```python
from build123d import *

# Parameters (mm, degrees)
EXTRUDE_1_DEPTH   = 2
HOLE_WIZARD_M81_D = 9
CHAMFER_1_SIZE    = 2


with BuildPart() as part:
    # Эскиз1 → Бобышка-Вытянуть1 (new body)
    with BuildSketch(Plane(origin=(0, 0, 0), x_dir=(1, 0, 0), z_dir=(0, 0, -1))):
        Polygon((0, 0), (0, 90), (90, 90), (90, 45), (45, 45), (45, 0), align=None)
    extrude(amount=EXTRUDE_1_DEPTH)

    # Отверстие с зазором M81 (through all)
    with Locations(Plane(origin=(0, 0, -2), x_dir=(1, 0, 0), z_dir=(0, 0, -1))):
        with Locations((22.5, 67.5), (22.5, 22.5), (67.5, 67.5)):
            Hole(HOLE_WIZARD_M81_D / 2)

    # Фаска1
    chamfer_1_edges = [part.edges().sort_by_distance(p)[0] for p in [
        (0, 0, -1),
        (0, -90, -1),
        (90, -90, -1),
        (90, -45, -1),
        (45, 0, -1),
    ]]
    chamfer(chamfer_1_edges, length=CHAMFER_1_SIZE)


solid = part.part
```
Verification items for the finished model (mm, model axes). A direction names the side the tool comes from. Round coordinates to 2 decimals unless told otherwise and drop trailing zeros. Loops run counter-clockwise (first coordinate to the right, second up) from the corner with the lowest first, then second, coordinate; pieces in that order, holes last. Notation, with made-up numbers: (33, -29.75) -> (89, -29.75) arc R11 cw to (89, -11.75) -> close; hole circle Ø10 at (40, 53). An arc over 180 degrees is marked (long way). Answer as a JSON object with one key per item and string values.
Q1. Draft check along Y on faces 3 (the flat face through (44, -1, -1)), 4 (the cylindrical face through (25.82, -25.54, -0.99)), 5 (the flat face through (45, -24, -1)). Enter one of: pulls with the +Y half, pulls with the -Y half, needs draft (parallel to the pull), parting line crosses it, or undercut.
Data:
{"face 3": "pulls with the +Y half", "face 4": "undercut", "face 5": "needs draft"}
Q2. Section check B-B (x = 67.5). Record the boundary of the cut face in (y, z), then the cut area to 3 significant figures.
Data:
{"outline": "(-90, -2) -> (-72, -2) -> (-72, 0) -> (-90, 0) -> close; (-63, -2) -> (-45, -2) -> (-45, 0) -> (-63, 0) -> close", "area": "72.0 mm2"}
Q3. Section check D-D (z = -1.2). Record the boundary of the cut face in (x, y), then the cut area to 3 significant figures.
Data:
{"outline": "(0, -88) -> (2, -90) -> (88, -90) -> (90, -88) -> (90, -47) -> (88, -45) -> (45, -45) -> (45, -2) -> (43, 0) -> (2, 0) -> (0, -2) -> close; hole circle Ø9 at (22.5, -67.5); hole circle Ø9 at (22.5, -22.5); hole circle Ø9 at (67.5, -67.5)", "area": "5,870 mm2"}
Q4. Section check C-C (y = -22.5). Record the boundary of the cut face in (x, z).
Data:
{"outline": "(0, -2) -> (18, -2) -> (18, 0) -> (0, 0) -> close; (27, -2) -> (45, -2) -> (45, 0) -> (27, 0) -> close"}
Q5. Access from +Z, -Z, +X, -X, +Y, -Y to the whole of each face (thin tool, end or side, straight path). Record for faces 1 (the flat face through (1, -89, -1)), 2 (the flat face through (67, -45, -1)).
Data:
{"face 1": "+Z, -Z, -X, -Y", "face 2": "+Z, -Z, +X, +Y"}
Q6. Section check A-A (x = 22.5). Record the boundary of the cut face in (y, z), then the cut area to 3 significant figures.
Data:
{"outline": "(-90, -2) -> (-72, -2) -> (-72, 0) -> (-90, 0) -> close; (-63, -2) -> (-27, -2) -> (-27, 0) -> (-63, 0) -> close; (-18, -2) -> (0, -2) -> (0, 0) -> (-18, 0) -> close", "area": "144 mm2"}
Q7. Go/stop test with flat-tipped pins: P1, Ø5.5, axis at x = 22.5, y = -22.5, coming from the +Z side; P2, Ø0.6, axis at y = -33, z = -1, coming from the +X side. Record where each tip stops, or that it passes through.
Data:
{"P1": "passes through", "P2": "stops at x = 45"}
Q8. Scan lines: line 1 (Y direction, x = 22.5, z = -0.5); line 2 (X direction, y = -67.5, z = -0.7); line 3 (Y direction, x = 67.5, z = -1.5). Record each from-to range of solid material in increasing order. Write a range as from..to.
Data:
{"line 1": "y = -90..-72, -63..-27, -18..0", "line 2": "x = 0..18, 27..63, 72..90", "line 3": "y = -90..-72, -63..-45"}
